```python
from build123d import *

# Parameters (mm, degrees)
BODY_DEPTH               = 6.35
CROSS_SUPPORT_REACH      = 170.123
SKETCH2_W                = 6.35
SKETCH2_H                = 30
SIDE_SUPPORTS_REACH      = 170.123
SKETCH3_W                = 6.35
SKETCH3_H                = 10
TOP_MOUNTING_TEETH_REACH = 170.123
SKETCH4_W                = 28.333333334
SKETCH4_H                = 6.35
LIGHTNING_HOLES_REACH    = 170.123


with BuildPart() as part:
    # Sketch1 → Body (new body)
    with BuildSketch(Plane.XY):
        Polygon((86.7, -50), (86.7, 0), (0, 0), (-50, 100), (-135, 100), (-135, -47), (0, -50), align=None)
    extrude(amount=BODY_DEPTH)

    # Sketch2 → Cross support (cut, up to next)
    with BuildSketch(Plane.XY.offset(6.35), mode=Mode.PRIVATE) as cross_support_sk1:
        with Locations((-131.825, -15)):
            Rectangle(SKETCH2_W, SKETCH2_H)
    cross_support_tool1 = extrude(cross_support_sk1.sketch, amount=-CROSS_SUPPORT_REACH, mode=Mode.PRIVATE) & part.part
    add(cross_support_tool1.solids().sort_by_distance((-131.825, -15, 6.35))[0], mode=Mode.SUBTRACT)

    # Sketch3 → Side supports (cut, up to next)
    with BuildSketch(Plane.XY.offset(6.35), mode=Mode.PRIVATE) as side_supports_sk1:
        with Locations((83.525, -15)):
            Rectangle(SKETCH3_W, SKETCH3_H)
    side_supports_tool1 = extrude(side_supports_sk1.sketch, amount=-SIDE_SUPPORTS_REACH, mode=Mode.PRIVATE) & part.part
    # Sketch3 → Side supports (cut, up to next)
    with BuildSketch(Plane.XY.offset(6.35), mode=Mode.PRIVATE) as side_supports_sk2:
        with Locations((83.525, -35)):
            Rectangle(SKETCH3_W, SKETCH3_H)
    side_supports_tool2 = extrude(side_supports_sk2.sketch, amount=-SIDE_SUPPORTS_REACH, mode=Mode.PRIVATE) & part.part
    # Sketch3 → Side supports (cut, up to next)
    with BuildSketch(Plane.XY.offset(6.35), mode=Mode.PRIVATE) as side_supports_sk3:
        with Locations((3.175, -35)):
            Rectangle(SKETCH3_W, SKETCH3_H)
    side_supports_tool3 = extrude(side_supports_sk3.sketch, amount=-SIDE_SUPPORTS_REACH, mode=Mode.PRIVATE) & part.part
    # Sketch3 → Side supports (cut, up to next)
    with BuildSketch(Plane.XY.offset(6.35), mode=Mode.PRIVATE) as side_supports_sk4:
        with Locations((3.175, -15)):
            Rectangle(SKETCH3_W, SKETCH3_H)
    side_supports_tool4 = extrude(side_supports_sk4.sketch, amount=-SIDE_SUPPORTS_REACH, mode=Mode.PRIVATE) & part.part
    add(side_supports_tool1.solids().sort_by_distance((83.525, -15, 6.35))[0], mode=Mode.SUBTRACT)
    add(side_supports_tool2.solids().sort_by_distance((83.525, -35, 6.35))[0], mode=Mode.SUBTRACT)
    add(side_supports_tool3.solids().sort_by_distance((3.175, -35, 6.35))[0], mode=Mode.SUBTRACT)
    add(side_supports_tool4.solids().sort_by_distance((3.175, -15, 6.35))[0], mode=Mode.SUBTRACT)

    # Sketch4 → Top mounting teeth (cut, up to next)
    with BuildSketch(Plane.XY.offset(6.35), mode=Mode.PRIVATE) as top_mounting_teeth_sk1:
        with Locations((-92.5, 96.825)):
            Rectangle(SKETCH4_W, SKETCH4_H)
    top_mounting_teeth_tool1 = extrude(top_mounting_teeth_sk1.sketch, amount=-TOP_MOUNTING_TEETH_REACH, mode=Mode.PRIVATE) & part.part
    # Sketch4 → Top mounting teeth (cut, up to next)
    with BuildSketch(Plane.XY.offset(6.35), mode=Mode.PRIVATE) as top_mounting_teeth_sk2:
        Polygon((-46.825, 93.65), (-50, 93.65), (-50, 100), align=None)
    top_mounting_teeth_tool2 = extrude(top_mounting_teeth_sk2.sketch, amount=-TOP_MOUNTING_TEETH_REACH, mode=Mode.PRIVATE) & part.part
    add(top_mounting_teeth_tool1.solids().sort_by_distance((-92.5, 96.825, 6.35))[0], mode=Mode.SUBTRACT)
    add(top_mounting_teeth_tool2.solids().sort_by_distance((-48.941667, 95.766667, 6.35))[0], mode=Mode.SUBTRACT)

    # Sketch6 → Lightning holes (cut, up to next)
    with BuildSketch(Plane.XY.offset(6.35), mode=Mode.PRIVATE) as lightning_holes_sk1:
        with BuildLine():
            Line((-118.65, 20), (-118.65, -20.886138472))
            ThreePointArc((-118.65, -20.886138472), (-116.114979028, -25.236296905), (-111.080448644, -25.175358194))
            Line((-111.080448644, -25.175358194), (-42.831323725, 15.710780278))
            ThreePointArc((-42.831323725, 15.710780278), (-40.581845168, 21.333023141), (-45.400875081, 25))
            Line((-45.400875081, 25), (-113.65, 25))
            ThreePointArc((-113.65, 25), (-117.185533906, 23.535533906), (-118.65, 20))
        make_face()
    lightning_holes_tool1 = extrude(lightning_holes_sk1.sketch, amount=-LIGHTNING_HOLES_REACH, mode=Mode.PRIVATE) & part.part
    # Sketch6 → Lightning holes (cut, up to next)
    with BuildSketch(Plane.XY.offset(6.35), mode=Mode.PRIVATE) as lightning_holes_sk2:
        with BuildLine():
            Line((-93.284496967, -37), (-25.035372048, -37))
            ThreePointArc((-25.035372048, -37), (-21.499838142, -35.535533906), (-20.035372048, -32))
            Line((-20.035372048, -32), (-20.035372048, 8.886138472))
            ThreePointArc((-20.035372048, 8.886138472), (-22.57039302, 13.236296905), (-27.604923404, 13.175358194))
            Line((-27.604923404, 13.175358194), (-95.854048323, -27.710780278))
            ThreePointArc((-95.854048323, -27.710780278), (-98.10352688, -33.333023141), (-93.284496967, -37))
        make_face()
    lightning_holes_tool2 = extrude(lightning_holes_sk2.sketch, amount=-LIGHTNING_HOLES_REACH, mode=Mode.PRIVATE) & part.part
    # Sketch6 → Lightning holes (cut, up to next)
    with BuildSketch(Plane.XY.offset(6.35), mode=Mode.PRIVATE) as lightning_holes_sk3:
        with BuildLine():
            Line((-125, 50.960581269), (-125, 78.65))
            ThreePointArc((-125, 78.65), (-123.535533906, 82.185533906), (-120, 83.65))
            Line((-120, 83.65), (-71.760111312, 83.65))
            ThreePointArc((-71.760111312, 83.65), (-66.928855022, 79.938007244), (-69.271034073, 74.313585064))
            Line((-69.271034073, 74.313585064), (-117.510922761, 46.624166333))
            ThreePointArc((-117.510922761, 46.624166333), (-122.505455428, 46.633608529), (-125, 50.960581269))
        make_face()
    lightning_holes_tool3 = extrude(lightning_holes_sk3.sketch, amount=-LIGHTNING_HOLES_REACH, mode=Mode.PRIVATE) & part.part
    # Sketch6 → Lightning holes (cut, up to next)
    with BuildSketch(Plane.XY.offset(6.35), mode=Mode.PRIVATE) as lightning_holes_sk4:
        with BuildLine():
            Line((-101.408826755, 44.336414936), (-53.168938067, 72.025833667))
            ThreePointArc((-53.168938067, 72.025833667), (-48.1744054, 72.016391471), (-45.679860828, 67.689418731))
            Line((-45.679860828, 67.689418731), (-45.679860828, 40))
            ThreePointArc((-45.679860828, 40), (-47.144326922, 36.464466094), (-50.679860828, 35))
            Line((-50.679860828, 35), (-98.919749516, 35))
            ThreePointArc((-98.919749516, 35), (-103.751005806, 38.711992756), (-101.408826755, 44.336414936))
        make_face()
    lightning_holes_tool4 = extrude(lightning_holes_sk4.sketch, amount=-LIGHTNING_HOLES_REACH, mode=Mode.PRIVATE) & part.part
    add(lightning_holes_tool1.solids().sort_by_distance((-89.16746, 6.594151, 6.35))[0], mode=Mode.SUBTRACT)
    add(lightning_holes_tool2.solids().sort_by_distance((-49.517912, -18.594151, 6.35))[0], mode=Mode.SUBTRACT)
    add(lightning_holes_tool3.solids().sort_by_distance((-102.306081, 69.637212, 6.35))[0], mode=Mode.SUBTRACT)
    add(lightning_holes_tool4.solids().sort_by_distance((-68.37378, 49.012788, 6.35))[0], mode=Mode.SUBTRACT)


solid = part.part
```
Model file for the job. Use its own axes, mm. A direction names the side the tool comes from. Coordinates: 2 decimals unless noted, no trailing zeros. Loops run counter-clockwise (first coordinate to the right, second up) from the corner with the lowest first, then second, coordinate; pieces in that order, holes last. Notation, with made-up numbers: M -4,78 L 50,78 A25 ccw 50,100 Z; hole C 34,72.5 d6. An arc over 180 degrees is marked long. Use CSV: the item, a comma, the result in double quotes. Start each with the question number.
1. Tool access for faces 5 (the flat face through (-93, 93.65, 3)), 6 (the flat face through (-74, 35, 3)), 7 (the flat face through (86.7, -45, 3)), 8 (the flat face through (83, -40, 3)): list every direction of +Z, -Z, +X, -X, +Y, -Y with a clear straight run to the whole face (end or side of a thin tool).
2. Band-saw the part on A-A, the plane y = -13. List the corners of the cut face in (x, z).
3. Probe probe 1 along X at (y, z) = (53, 2.25); probe 2 along Y at (x, z) = (-91.5, 2); probe 3 along Y at (x, z) = (-107, 2.5). List the from-to ranges inside material, lowest first. Write a range as [from, to].
4. Band-saw the part on C-C, the plane z = 2.5. Give the number of separate pieces and of enclosed holes in the cut face, then the cut area to 3 significant figures.
5. Two-plate mould, pull along X, no slides. Class faces 1 (the flat face through (83, -10, 3)), 2 (the flat face through (-128.65, -15, 3)), 3 (the flat face through (86.7, -5, 3)), 4 (the flat face through (3, -30, 3)): pulls with the +X half, pulls with the -X half, needs draft (parallel to the pull), parting line crosses it, or undercut.
6. Flat gauge pins, fed straight in: pin 1 (1.9 mm diameter, centred on y = -13.5, z = 4, fed in from +X); pin 2 (3 mm diameter, centred on y = 52.5, z = 5, fed in from +X); pin 3 (3 mm diameter, centred on x = 2.5, z = 3.5, fed in from +Y). Where does each tip first touch, or does it go through?
7. Band-saw the part on D-D, the plane x = 16. List the corners of the cut face in (y, z).
8. Band-saw the part on B-B, the plane x = -31. List the corners of the cut face in (y, z).
Entries:
1,face 5,"+Z, -Z, +Y"
1,face 6,"+Z, -Z"
1,face 7,"+Z, -Z, +X, +Y, -Y"
1,face 8,"+Z, -Z, +X"
2,outline,"M -128.65,0 L -118.65,0 L -118.65,6.35 L -128.65,6.35 Z; M -90.76,0 L -71.3,0 L -71.3,6.35 L -90.76,6.35 Z; M -20.04,0 L 0,0 L 0,6.35 L -20.04,6.35 Z; M 6.35,0 L 80.35,0 L 80.35,6.35 L 6.35,6.35 Z"
3,probe 1,"x = [-135, -125], [-106.4, -86.32], [-45.68, -26.5]"
3,probe 2,"y = [-47.97, -37], [-25.1, -13.45], [25, 35], [50.02, 61.55], [83.65, 93.65]"
3,probe 3,"y = [-47.62, -22.73], [25, 52.66], [83.65, 100]"
4,separate pieces,"1"
4,enclosed holes,"6"
4,area,"13,600 mm2"
5,face 1,"needs draft"
5,face 2,"pulls with the -X half"
5,face 3,"pulls with the +X half"
5,face 4,"undercut"
6,pin 1,"stops at x = 80.35"
6,pin 2,"stops at x = -25.5"
6,pin 3,"stops at y = 0"
7,outline,"M -50,0 L 0,0 L 0,6.35 L -50,6.35 Z"
8,outline,"M -49.31,0 L -37,0 L -37,6.35 L -49.31,6.35 Z; M 11.14,0 L 62,0 L 62,6.35 L 11.14,6.35 Z"
